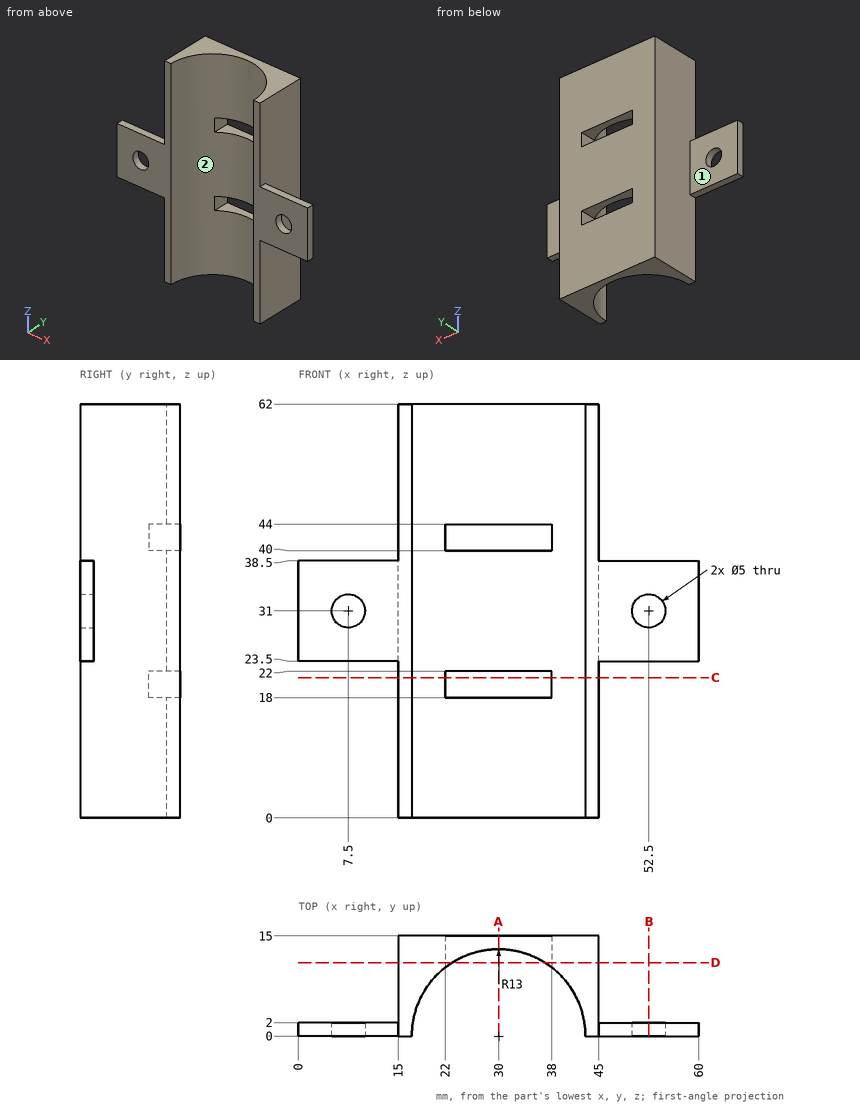
Job drawing, mm, ordinate dimensions from the low corner. One solid piece. Coordinates: 2 decimals unless noted, no trailing zeros. Write each loop counter-clockwise with the first axis right and the second up, starting at its lowest first coordinate (ties: lowest second). Pieces come first, ordered by that corner, then holes. Notation, with made-up numbers: (89.25, 26.25) - (144.25, 26.25) arc R15 ccw to (144.25, 50.25) - close; hole circle Ø6 at (38.25, -30.75). An arc over 180 degrees is marked (long way). Use a Markdown table: item, result. Add a question column.
Item 1: Band-saw the part on B-B, the plane x = 52.5. Give the cut face in (y, z), and give its area (3 significant figures).
Item 2: Band-saw the part on D-D, the plane y = 11. Give the cut face in (x, z), and give its area (3 significant figures).
Item 3: Band-saw the part on A-A, the plane x = 30. Give the cut face in (y, z).
Item 4: Drill centre lines: L1, parallel to X at y = 0.65, z = 31; L2, parallel to Z at x = 52.5, y = 1.5; L3, parallel to X at y = 1.5, z = 31. Where is each one in solid material? Low to high. Write a range as from..to.
Item 5: Mould opens along X. For the marked faces 1 and 2 say: pulls with the +X half, pulls with the -X half, needs draft (parallel to the pull), parting line crosses it, or undercut.
Item 6: Flat gauge pins, fed straight in: pin 1 (1.2 mm diameter, centred on y = 12.5, z = 41.5, fed in from -X); pin 2 (1 mm diameter, centred on x = 49, y = 1, fed in from -Z); pin 3 (3 mm diameter, centred on y = 12.5, z = 41.5, fed in from +X). Where does each tip first touch, or does it go through?
Item 7: Band-saw the part on C-C, the plane z = 21. Give the cut face in (x, y).
Numbers:
| question | item | result |
|---|---|---|
| 1 | outline | (0, 23.5) - (2, 23.5) - (2, 28.5) - (0, 28.5) - close; (0, 33.5) - (2, 33.5) - (2, 38.5) - (0, 38.5) - close |
| 1 | area | 20.0 mm2 |
| 2 | outline | (15, 0) - (23.07, 0) - (23.07, 18) - (22, 18) - (22, 22) - (23.07, 22) - (23.07, 40) - (22, 40) - (22, 44) - (23.07, 44) - (23.07, 62) - (15, 62) - close; (36.93, 0) - (45, 0) - (45, 62) - (36.93, 62) - (36.93, 44) - (38, 44) - (38, 40) - (36.93, 40) - (36.93, 22) - (38, 22) - (38, 18) - (36.93, 18) - close |
| 2 | area | 984 mm2 |
| 3 | outline | (13, 0) - (15, 0) - (15, 18) - (13, 18) - close; (13, 22) - (15, 22) - (15, 40) - (13, 40) - close; (13, 44) - (15, 44) - (15, 62) - (13, 62) - close |
| 4 | L1 | 0..5, 10..17.02, 42.98..50, 55..60 |
| 4 | L2 | 23.5..28.5, 33.5..38.5 |
| 4 | L3 | 0..5, 10..17.09, 42.91..50, 55..60 |
| 5 | face 1 | needs draft |
| 5 | face 2 | undercut |
| 6 | pin 1 | x = 15 |
| 6 | pin 2 | z = 23.5 |
| 6 | pin 3 | x = 45 |
| 7 | outline | (15, 0) - (17, 0) arc R13 cw to (22, 10.25) - (22, 15) - (15, 15) - close; (38, 10.25) arc R13 cw to (43, 0) - (45, 0) - (45, 15) - (38, 15) - close |
